The listing builds one solid part. Answer for the finished solid, in the listing's coordinates (mm). A direction names the side the tool comes from. Round coordinates to 2 decimals unless told otherwise and drop trailing zeros. Write each loop counter-clockwise with the first axis right and the second up, starting at its lowest first coordinate (ties: lowest second). Pieces come first, ordered by that corner, then holes. Notation, with made-up numbers: (39, 73.25) - (49, 73.25) arc R25 ccw to (49, 94.25) - close; hole circle Ø8 at (-18.75, -13.5). An arc over 180 degrees is marked (long way). Answer as CSV lines item,"result". Start each with the question number.
Item 1: For a pull along Z with two mould halves and no side action, classify faces 6 (the flat face through (92, 42, 18)), 7 (the flat face through (44, 2, 30)), 8 (the cylindrical face through (93.52, 22.1, 12.07)) as pulls with the +Z half, pulls with the -Z half, needs draft (parallel to the pull), parting line crosses it, or undercut.
Item 2: A cutting plane is placed at D-D on y = 10. Determine the outline of the cut face in (x, z), and give its area (3 significant figures).
Item 3: Which of the six approach directions +Z, -Z, +X, -X, +Y, -Y give full straight-line access (tool end or side, diameter ignored) to faces 1 (the flat face through (1, 64, 15)), 2 (the flat face through (47, 23, 3)), 3 (the cylindrical face through (93.521, 59.253, 15.132)), 4 (the flat face through (95, 42, 15)), 5 (the flat face through (47, 43, 0))?
Item 4: A cutting plane is placed at C-C on x = 42. Determine the outline of the cut face in (y, z).
Item 5: Straight lines are drawn through the part: line 1 along X through (y, z) = (67, 18.25); line 2 along Y through (x, z) = (75, 20.75); line 3 along Z through (x, y) = (93.8, 62.25). For each, find the intervals that lie inside material, in ascending order. Write a range as [from, to].
Item 6: A cutting plane is placed at B-B on y = 62.25. Determine the outline of the cut face in (x, z), and give its area (3 significant figures).
Item 7: Flat-ended cylindrical pins translate along their axes: pin 1 (23.5 mm diameter, centred on x = 63.5, y = 26, fed in from +Z); pin 2 (1 mm diameter, centred on y = 66.5, z = 6.5, fed in from -X); pin 3 (3.5 mm diameter, centred on y = 22.75, z = 15, fed in from +X). Find the tip coordinate at first contact, or state that the pin passes through.
Item 8: A cutting plane is placed at A-A on z = 6.25. Determine the outline of the cut face in (x, y), and give its area (3 significant figures).
```python
from build123d import *

# Parameters (mm, degrees)
SKETCH_W        = 95
SKETCH_H        = 85
EXTRUDE_DEPTH   = 30
SKETCH002_W     = 89
SKETCH002_H     = 79
POCKET_DEPTH    = 25
SKETCH001_W     = 85
SKETCH001_H     = 35
POCKET001_DEPTH = 27
SKETCH003_R     = 3
HOLE_DEPTH      = 25
HOLE_TIPS_R     = 3
SKETCH004_W     = 18.43
SKETCH004_H     = 5
POCKET002_DEPTH = 3


with BuildPart() as part:
    # Sketch → Extrude (new body)
    with BuildSketch(Plane.XY):
        with Locations((47.5, 42.5)):
            Rectangle(SKETCH_W, SKETCH_H)
    extrude(amount=EXTRUDE_DEPTH)

    # Sketch002 (on Face6 of BaseFeature) → Pocket (cut)
    with BuildSketch(Plane.XY.offset(30)):
        with Locations((47.5, 42.5)):
            Rectangle(SKETCH002_W, SKETCH002_H)
    extrude(amount=-POCKET_DEPTH, mode=Mode.SUBTRACT)

    # Sketch001 (on Face6 of BaseFeature) → Pocket001 (cut)
    with BuildSketch(Plane.XY.offset(30)):
        with Locations((47.5, 62.644853)):
            Rectangle(SKETCH001_W, SKETCH001_H)
        with Locations((47.5, 22.5)):
            Rectangle(SKETCH001_W, SKETCH001_H)
    extrude(amount=-POCKET001_DEPTH, mode=Mode.SUBTRACT)

    # Sketch003 (on Face3 of Pocket001) → Hole (cut)
    with BuildSketch(Plane.YZ.offset(95)):
        with Locations((22.75, 15)):
            Circle(SKETCH003_R)
        with Locations((62.25, 15)):
            Circle(SKETCH003_R)
    extrude(amount=-HOLE_DEPTH, mode=Mode.SUBTRACT)

    # Hole tips → Hole tip 1 section 0
    with BuildSketch(Plane.YZ.offset(70), mode=Mode.PRIVATE) as hole_tip_1_s0:
        with Locations((22.75, 15)):
            Circle(HOLE_TIPS_R)
    loft([hole_tip_1_s0.sketch, Vertex(68.197418, 22.75, 15)], mode=Mode.SUBTRACT)

    # Hole tips → Hole tip 2 section 0
    with BuildSketch(Plane.YZ.offset(70), mode=Mode.PRIVATE) as hole_tip_2_s0:
        with Locations((62.25, 15)):
            Circle(HOLE_TIPS_R)
    loft([hole_tip_2_s0.sketch, Vertex(68.197418, 62.25, 15)], mode=Mode.SUBTRACT)

    # Sketch004 (on Face2 of Hole) → Pocket002 (cut)
    with BuildSketch(Plane(origin=(0, 0, 0), x_dir=(0, -1, 0), z_dir=(-1, 0, 0))):
        with Locations((-63.57, 12.5)):
            Rectangle(SKETCH004_W, SKETCH004_H)
        with Locations((-21.425, 12.5)):
            Rectangle(SKETCH004_W, SKETCH004_H)
    extrude(amount=-POCKET002_DEPTH, mode=Mode.SUBTRACT)


solid = part.part
```
Geometry says:
1,face 6,"needs draft"
1,face 7,"pulls with the +Z half"
1,face 8,"undercut"
2,outline,"(0, 0) - (95, 0) - (95, 30) - (92, 30) - (92, 5) - (90, 5) - (90, 3) - (5, 3) - (5, 5) - (3, 5) - (3, 30) - (0, 30) - close"
2,area,"455 mm^2"
3,face 1,"-X"
3,face 2,"+Z"
3,face 3,"+X"
3,face 4,"+Z, -Z, +X, +Y, -Y"
3,face 5,"-Z, +X, -X, +Y, -Y"
4,outline,"(0, 0) - (85, 0) - (85, 30) - (82, 30) - (82, 5) - (80.14, 5) - (80.14, 3) - (45.14, 3) - (45.14, 5) - (40, 5) - (40, 3) - (5, 3) - (5, 5) - (3, 5) - (3, 30) - (0, 30) - close"
5,line 1,"x = [0, 3], [92, 95]"
5,line 2,"y = [0, 3], [82, 85]"
5,line 3,"z = [0, 12], [18, 30]"
6,outline,"(0, 0) - (95, 0) - (95, 12) - (92, 12) - (92, 5) - (90, 5) - (90, 3) - (5, 3) - (5, 5) - (3, 5) - (3, 10) - (0, 10) - close; (0, 15) - (3, 15) - (3, 30) - (0, 30) - close; (92, 18) - (95, 18) - (95, 30) - (92, 30) - close"
6,area,"422 mm^2"
7,pin 1,"stops at z = 3"
7,pin 2,"stops at x = 0"
7,pin 3,"stops at x = 3"
8,outline,"(0, 0) - (95, 0) - (95, 85) - (0, 85) - close; hole (3, 3) - (92, 3) - (92, 82) - (3, 82) - close"
8,area,"1,040 mm^2"
